```python
from build123d import *

# Parameters (mm, degrees)
PATTERN_LINEAR_1_COUNT = 3
PATTERN_LINEAR_1_PITCH = 25.5
CHAMFER_1_SIZE         = 1
SKETCH_4_W             = 20
SKETCH_4_H             = 6.257919358
CUT_EXTRUDE_1_DEPTH    = 202.457390036


with BuildPart() as part:
    # 草图1 → 旋转1 (revolve)
    with BuildSketch(Plane.XY, mode=Mode.PRIVATE) as revolve_1_sk:
        Polygon((0, 37.5), (0, 129.8), (83, 129.8), (83, 62.5), (50, 62.5), (50, 37.5), align=None)
    revolve(revolve_1_sk.sketch.rotate(Axis((0, 0, 0), (1, 0, 0)), 90), axis=Axis((0, 0, 0), (1, 0, 0)))

    # 草图2 → 切除-旋转1 (revolve, cut)
    with BuildSketch(Plane.XY, mode=Mode.PRIVATE) as cut_revolve_1_sk:
        Polygon((21.128051255, 110.7), (26.967507271, 129.8), (5.032492729, 129.8), (10.871948745, 110.7), align=None)
    cut_revolve_1 = revolve(cut_revolve_1_sk.sketch.rotate(Axis((0, 0, 0), (1, 0, 0)), 90), axis=Axis((0, 0, 0), (1, 0, 0)), mode=Mode.SUBTRACT)

    # 阵列(线性)1: 切除-旋转1 ×3
    with Locations(*[(i * PATTERN_LINEAR_1_PITCH, 0, 0) for i in range(1, PATTERN_LINEAR_1_COUNT)]):
        add(cut_revolve_1, mode=Mode.SUBTRACT)

    # 倒角1
    chamfer_1_edges = [part.edges().sort_by_distance(p)[0] for p in [
        (0, 0, -37.5),
        (50, 0, -37.5),
    ]]
    chamfer(chamfer_1_edges, length=CHAMFER_1_SIZE)

    # 草图4 → 切除-拉伸1 (cut, through all)
    with BuildSketch(Plane.ZY):
        with Locations((0, 39.271040416)):
            Rectangle(SKETCH_4_W, SKETCH_4_H)
    extrude(amount=-CUT_EXTRUDE_1_DEPTH, mode=Mode.SUBTRACT)


solid = part.part
```
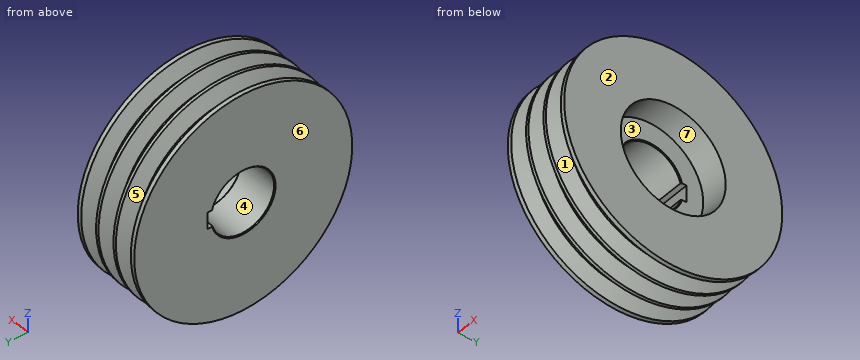
The listing builds one solid part. Answer for the finished solid, in the listing's coordinates (mm). Face numbers are marked on the shaded views. A direction names the side the tool comes from. Round coordinates to 2 decimals unless told otherwise and drop trailing zeros. Return JSON: item names as keys, results as strings. Group by question number.
1. The mould has two halves that part along Y. Classify the marked faces 1, 2, 3 and 4: pulls with the +Y half, pulls with the -Y half, needs draft (parallel to the pull), parting line crosses it, or undercut.
2. Consider probe 1 along X at (y, z) = (14, -110); probe 2 along X at (y, z) = (114, -57); probe 3 along X at (y, z) = (38, 30.5). Determine where each line is inside the solid, lowest interval first.
3. Which of the six approach directions +Z, -Z, +X, -X, +Y, -Y give full straight-line access (tool end or side, diameter ignored) to the marked faces 5, 6 and 7?
4. Each of these flat-tipped pins is pushed along its axis until it touches: P1, Ø5, axis at x = 51.5, z = 9.5, coming from the +Y side; P2, Ø1.5, axis at x = 40.5, z = 56, coming from the +Y side; P3, Ø3, axis at x = 14.5, y = -34, coming from the +Z side. Where does it stop, or does it pass through?
Resolved:
{
 "1": {"face 1": "parting line crosses it", "face 2": "needs draft", "face 3": "undercut", "face 4": "undercut"},
 "2": {"probe 1": "x = 0 to 10.81, 21.19 to 36.31, 46.69 to 61.81, 72.19 to 83", "probe 2": "x = 0 to 5.75, 26.25 to 31.25, 51.75 to 56.75, 77.25 to 83", "probe 3": "x = 0 to 50"},
 "3": {"face 5": "none", "face 6": "+Z, -Z, -X, +Y, -Y", "face 7": "+X"},
 "4": {"P1": "stops at y = 129.6", "P2": "stops at y = 95.93", "P3": "stops at z = 105.82"}
}
